CAD build for the part. Positions are in the model's coordinates, mm. Round coordinates to 2 decimals unless told otherwise and drop trailing zeros. Loops run counter-clockwise (first coordinate to the right, second up) from the corner with the lowest first, then second, coordinate; pieces in that order, holes last.
Autodesk Inventor part; units mm, degrees
ref_plane "YZ Plane" through (0, 0, 0) normal (1, 0, 0) x (0, 1, 0)
ref_plane "XZ Plane" through (0, 0, 0) normal (0, 1, 0) x (-1, 0, 0)
ref_plane "XY Plane" through (0, 0, 0) normal (0, 0, 1) x (1, 0, 0)
sketch "Sketch1" plane through (0, 0, 0) normal (0, 0, 1) x (1, 0, 0)
  arc A0 (214.793, 155.575) -> (-1.2995, -306.5385) centre (-54.6708, 0) ccw
  line L0 (-1.2995, -306.5385) -> (-100.7285, -323.85)
  line L1 (-189.1562, -406.4) -> (313.6292, -406.4)
  line L2 (351.7292, -406.4) -> (351.7292, 0)
  arc A1 (-1.2995, -306.5385) -> (214.793, 155.575) centre (-54.6708, 0) ccw
  line L3 (-54.6708, 0) -> (401.7178, 0) construction
  arc A2 (351.7292, 0) -> (297.2819, 203.2) centre (-54.6708, 0) ccw
  line L4 (297.2819, 203.2) -> (214.793, 155.575)
  line L5 (34.2292, -406.4) -> (59.6292, -406.4)
  line L6 (59.6292, -406.4) -> (59.6292, -381)
  line L7 (59.6292, -381) -> (34.2292, -381)
  line L8 (34.2292, -381) -> (34.2292, -406.4)
  line L9 (288.2292, -406.4) -> (351.7292, -406.4)
  line L10 (313.6292, -406.4) -> (313.6292, -381)
  line L11 (313.6292, -381) -> (288.2292, -381)
  line L12 (288.2292, -381) -> (288.2292, -406.4)
  circle A3 centre (-54.6708, 0) radius 200.5558 construction
  line L13 (313.6292, 12.7) -> (339.0292, 12.7)
  line L14 (339.0292, 12.7) -> (339.0292, -12.7)
  line L15 (339.0292, -12.7) -> (313.6292, -12.7)
  line L16 (313.6292, -12.7) -> (313.6292, 12.7)
  line L17 (313.6292, 12.7) -> (339.0292, -12.7) construction
  line L18 (339.0292, 12.7) -> (313.6292, -12.7) construction
  line L19 (-189.1562, -406.4) -> (-358.8569, -425.45)
  line L20 (-358.8569, -425.45) -> (351.7292, -425.45)
  line L21 (351.7292, -425.45) -> (351.7292, -406.4)
  line L22 (313.6292, -406.4) -> (351.7292, -406.4)
  line L23 (-358.8569, -425.45) -> (-100.7285, -323.85)
  line L24 (-100.7285, -323.85) -> (-227.7285, -323.85)
  line L25 (-227.7285, -323.85) -> (-460.4569, -425.45)
  line L26 (-460.4569, -425.45) -> (-358.8569, -425.45)
  line L27 (-245.1708, -381) -> (-219.7708, -381)
  line L28 (-219.7708, -381) -> (-219.7708, -406.4)
  line L29 (-219.7708, -406.4) -> (-245.1708, -406.4)
  line L30 (-245.1708, -406.4) -> (-245.1708, -381)
  line L31 (-100.7285, -323.85) -> (-189.1562, -406.4)
  point P0 (290.2482, -355.6)
  point P1 (326.3292, 0)
  point P2 (326.3292, 0)
  point P3 (302.9482, -330.2)
  point P4 (298.4754, -355.6)
  point P5 (302.9482, -12.7)
  point P6 (302.7291, 12.7)
  point P7 (-245.1708, -386.8886)
  point P8 (-227.8836, -381)
  dimension "d0" = 622.3
  dimension "d1" = 406.4
  dimension "d2" = 30
  dimension "d4" = 406.4
  dimension "d7" = 25.4
  dimension "d8" = 25.4
  dimension "d9" = 38.1
  dimension "d10" = 292.1
  dimension "d21" = 25.4
  dimension "d22" = 25.4
  dimension "d23" = 25.4
  dimension "d27" = 19.05
  dimension "d32" = 101.6
  dimension "d33" = 101.6
  dimension "d40" = 254
  dimension "d41" = 127
extrude "Extrusion1" add sketch "Sketch1" along normal blind 12.7 contours L4 A2 L2 L9 L10 L11 L12 L1 L6 L7 L8 L31 L0 A1 | L31 L19 L23 | L23 L26 L25 L24 | L19 L1 L9 L21 L20
ref_plane "Work Plane1" through (59.6292, 0, 0) normal (0, 1, 0) x (-1, 0, 0)
fillet "Fillet3" radius 127 2 edges at (-100.7285, -323.85, 6.35) (-227.7285, -323.85, 6.35)
fillet "Fillet3" radius 6.35 1 edges at (-460.4569, -425.45, 6.35)
sketch "Sketch3" plane through (59.6292, 0, 0) normal (0, 1, 0) x (-1, 0, 0)
  line L0 (314.8558, -44.45) -> (-86.2558, -44.45) construction
  line L1 (114.3, -44.45) -> (114.3, -0.9544) construction
  circle A0 centre (355.6, -69.85) radius 88.9
  point P0 (59.6292, 0)
  dimension "d17" = 25.4
  dimension "d18" = 177.8
  dimension "d19" = 241.3
revolve "Revolution2" cut sketch "Sketch3" angle 360 about axis through (-54.6708, 0, -44.45) along (0, 0, 1)
sketch "Sketch4" plane through (0, 0, 12.7) normal (0, 0, 1) x (1, 0, 0)
  circle A0 centre (85.0292, -393.7) radius 3.3734
  circle A1 centre (104.0792, -393.7) radius 3.3734
  circle A2 centre (123.1292, -393.7) radius 3.3734
  circle A3 centre (224.7292, -393.7) radius 3.3734
  circle A4 centre (243.7792, -393.7) radius 3.3734
  circle A5 centre (262.8292, -393.7) radius 3.3734
  circle A6 centre (300.9292, -355.6) radius 3.3734
  circle A7 centre (300.9292, -336.55) radius 3.3734
  circle A8 centre (300.9292, -317.5) radius 3.3734
  circle A9 centre (326.3292, -76.2) radius 3.3734
  circle A10 centre (326.3292, -57.15) radius 3.3734
  circle A11 centre (326.3292, -38.1) radius 3.3734
  circle A12 centre (-156.2708, -393.7) radius 3.3734
  circle A13 centre (-175.3208, -393.7) radius 3.3734
  circle A14 centre (-194.3708, -393.7) radius 3.3734
  point P0 (0, 0)
extrude "Extrusion2" cut sketch "Sketch4" against normal through all
sketch "Sketch5" plane through (0, 0, 12.7) normal (0, 0, 1) x (1, 0, 0)
  line L0 (351.7292, -425.45) -> (314.3912, -425.45)
  line L1 (314.3912, -425.45) -> (314.3912, -328.676)
  line L2 (314.3912, -328.676) -> (351.7292, -328.676)
  line L3 (351.7292, -328.676) -> (351.7292, -425.45)
  line L4 (314.3912, -331.851) -> (314.3912, -328.676)
  point P0 (0, 0)
extrude "Extrusion3" cut sketch "Sketch5" against normal through all
properties part number "OuterWheelIndexer"
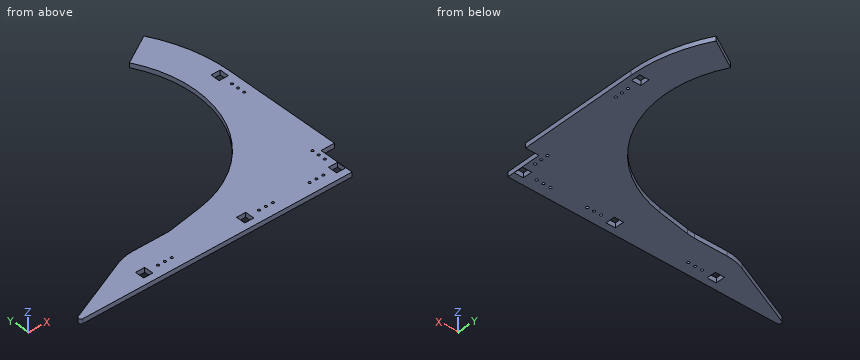
Item 1: Flat gauge pins, fed straight in: P1, Ø11, axis at x = -156.27, y = -393.7, coming from the +Z side; P2, Ø5, axis at y = 27, z = 7.5, coming from the +X side; P3, Ø4, axis at x = -328, z = 10, coming from the +Y side; P4, Ø4, axis at x = 44.5, z = 5, coming from the +Y side. Where does each tip first touch, or does it go through?
Answers follow:
P1: stops at z = 12.7
P2: stops at x = 350.99
P3: stops at y = -366.75
P4: stops at y = -294.24
Item 2: Cut at C-C, the plane y = -233.5. Give the cut face in (x, z), plus the area to 3 significant figures.
Answers follow:
outline: (150.98, 0) - (351.73, 0) - (351.73, 12.7) - (150.98, 12.7) - close
area: 2,550 mm2
Item 3: Cut at B-B, the plane x = -14. Give the cut face in (y, z).
Answers follow:
outline: (-425.45, 0) - (-308.75, 0) - (-308.75, 12.7) - (-425.45, 12.7) - close
Item 4: Cut at A-A, the plane z = 9.5. State how many separate pieces and enclosed holes the cut face has, plus the area to 3 significant figures.
Answers follow:
separate pieces: 1
enclosed holes: 19
area: 137,000 mm2
Item 5: Probe line 1 (Y direction, x = -190.5, z = 2); line 2 (Y direction, x = -0.5, z = 5); line 3 (Y direction, x = 123.5, z = 3). List the from-to ranges inside material, lowest first.
Answers follow:
line 1: y = -425.45 to -323.85
line 2: y = -425.45 to -306.4
line 3: y = -425.45 to -397.05, -390.35 to -255.09
